Input: part model. Units: mm. Frame: model coordinates. Give positions to 0.01 mm unless a question says otherwise; leave off trailing zeros. Write each loop counter-clockwise with the first axis right and the second up, starting at its lowest first coordinate (ties: lowest second). Pieces come first, ordered by that corner, then holes. Notation, with made-up numbers: (43, 21.25) -> (57, 21.25) arc R34 cw to (57, 60.25) -> close; hole circle Ø9 at (10.25, 83.5). An arc over 180 degrees is marked (long way). Return JSON: item names as keys, results as strings. Group by question number.
Item 1: Section C-C, the plane z = 113.5. Return loops of the section in (x, y), then the cut area to 3 significant figures.
Item 2: Line query: line 1 (X direction, y = 11.5, z = -37) (3 decimals); line 2 (Z direction, x = 33, y = 10.5); line 3 (X direction, y = 0.5, z = 22.5). Output: solid intervals per line, ascending. Write a range as [from, to].
Item 3: Section A-A, the plane y = 9.25. Count the separate pieces of the cut face and the enclosed holes in it, then the cut area to 3 significant figures.
Item 4: Pin query (flat end, axial travel): P1, Ø4, axis at y = 6.5, z = 48.5, coming from the +X side; P2, Ø6.5, axis at x = 586.5, y = 7.5, coming from the +Z side; P3, Ø4, axis at y = 7, z = 96, coming from the -X side. Return the tip coordinate at first contact, or that it passes through.
Item 5: Section B-B, the plane x = 58. Return loops of the section in (y, z).
from build123d import *

# Parameters (mm, degrees)
BOSS_EXTRUDE1_DEPTH = 12.7


with BuildPart() as part:
    # Sketch1 → Boss-Extrude1 (new body)
    with BuildSketch(Plane(origin=(0, 0, 0), x_dir=(1, 0, 0), z_dir=(0, 1, 0))):
        Polygon((0, 0), (96.04375, 0), (96.04375, -190.5), (559.59375, -190.5), (559.59375, 0), (606.425, 0), (606.425, 819.15), (0, 819.15), align=None)
        with BuildLine():
            Line((19.05, 41.4782), (31.75, 41.4782))
            ThreePointArc((31.75, 41.4782), (35.1282, 38.1), (31.75, 34.7218))
            Line((31.75, 34.7218), (19.05, 34.7218))
            ThreePointArc((19.05, 34.7218), (15.6718, 38.1), (19.05, 41.4782))
        make_face(mode=Mode.SUBTRACT)
        with BuildLine():
            Line((19.05, 441.5282), (31.75, 441.5282))
            ThreePointArc((31.75, 441.5282), (35.1282, 438.15), (31.75, 434.7718))
            Line((31.75, 434.7718), (19.05, 434.7718))
            ThreePointArc((19.05, 434.7718), (15.6718, 438.15), (19.05, 441.5282))
        make_face(mode=Mode.SUBTRACT)
        with BuildLine():
            Line((31.75, 784.0218), (19.05, 784.0218))
            ThreePointArc((19.05, 784.0218), (15.6718, 787.4), (19.05, 790.7782))
            Line((19.05, 790.7782), (31.75, 790.7782))
            ThreePointArc((31.75, 790.7782), (35.1282, 787.4), (31.75, 784.0218))
        make_face(mode=Mode.SUBTRACT)
        with BuildLine():
            Line((577.85, 784.0218), (590.55, 784.0218))
            ThreePointArc((590.55, 784.0218), (593.9282, 787.4), (590.55, 790.7782))
            Line((590.55, 790.7782), (577.85, 790.7782))
            ThreePointArc((577.85, 790.7782), (574.4718, 787.4), (577.85, 784.0218))
        make_face(mode=Mode.SUBTRACT)
        with BuildLine():
            Line((590.55, 441.5282), (577.85, 441.5282))
            ThreePointArc((577.85, 441.5282), (574.4718, 438.15), (577.85, 434.7718))
            Line((577.85, 434.7718), (590.55, 434.7718))
            ThreePointArc((590.55, 434.7718), (593.9282, 438.15), (590.55, 441.5282))
        make_face(mode=Mode.SUBTRACT)
        with BuildLine():
            Line((590.55, 41.4782), (577.85, 41.4782))
            ThreePointArc((577.85, 41.4782), (574.4718, 38.1), (577.85, 34.7218))
            Line((577.85, 34.7218), (590.55, 34.7218))
            ThreePointArc((590.55, 34.7218), (593.9282, 38.1), (590.55, 41.4782))
        make_face(mode=Mode.SUBTRACT)
    extrude(amount=BOSS_EXTRUDE1_DEPTH)


solid = part.part
Answer below:
{
 "1": {"outline": "(96.04, 0) -> (559.59, 0) -> (559.59, 12.7) -> (96.04, 12.7) -> close", "area": "5,890 mm2"},
 "2": {"line 1": "x = [0, 15.856], [34.944, 574.656], [593.744, 606.425]", "line 2": "z = [-819.15, -790.54], [-784.26, -441.29], [-435.01, -41.24], [-34.96, 0]", "line 3": "x = [96.04, 559.59]"},
 "3": {"separate pieces": "1", "enclosed holes": "6", "area": "584,000 mm2"},
 "4": {"P1": "stops at x = 559.59", "P2": "stops at z = 0", "P3": "stops at x = 96.04"},
 "5": {"outline": "(0, -819.15) -> (12.7, -819.15) -> (12.7, 0) -> (0, 0) -> close"}
}
